from build123d import *

# Parameters (mm, degrees)
SKETCH_2_R                   = 2.5
SM_BASE_FLANGE_1_DEPTH       = 2
FILLET_1_R                   = 5
SM_EDGE_FLANGE_1_DEPTH       = 105
SM_EDGE_FLANGE_2_DEPTH       = 65
SM_START                     = 2
SM_EDGE_FLANGE_2_PROFILE_W   = 65
SM_EDGE_FLANGE_2_PROFILE_H   = 131
SM_EDGE_FLANGE_2_PROFILE_W_2 = 28
SM_EDGE_FLANGE_2_PROFILE_H_2 = 3
SM_EDGE_FLANGE_2_FLAT_DEPTH  = 2
SM_EDGE_FLANGE_3_DEPTH       = 105
SM_EDGE_FLANGE_3_PROFILE_W   = 9
SM_EDGE_FLANGE_3_PROFILE_H   = 9
SM_EDGE_FLANGE_3_FLAT_DEPTH  = 2
FILLET_3_R                   = 5
FILLET_4_R                   = 2
SM_EDGE_FLANGE_4_DEPTH       = 50
SM_EDGE_FLANGE_4_BEND_DEPTH  = 50
FILLET_2_R                   = 10


# Sheet-metal steps are written as plain solids
with BuildPart() as part:
    # Sketch 2 → Базовая кромка1 (new body)
    with BuildSketch(Plane(origin=(0, 0, 0), x_dir=(1, 0, 0), z_dir=(0, 1, 0))):
        Polygon((-90, -54), (-90, -86), (90, -86), (90, -66), (105, -66), (105, -34), (90, -34), (90, 34), (105, 34), (105, 66), (90, 66), (90, 86), (-90, 86), (-90, 54), (-75, 54), (-75, -54), align=None)
        with Locations(Location((-83, 80, 0), (0, 0, 270))):
            Circle(SKETCH_2_R, mode=Mode.SUBTRACT)
        with Locations(Location((-83, 60, 0), (0, 0, 270))):
            Circle(SKETCH_2_R, mode=Mode.SUBTRACT)
        with Locations(Location((98, 60, 0), (0, 0, 270))):
            Circle(SKETCH_2_R, mode=Mode.SUBTRACT)
        with Locations(Location((98, 40, 0), (0, 0, 270))):
            Circle(SKETCH_2_R, mode=Mode.SUBTRACT)
        with Locations(Location((98, -40, 0), (0, 0, 270))):
            Circle(SKETCH_2_R, mode=Mode.SUBTRACT)
        with Locations(Location((98, -60, 0), (0, 0, 270))):
            Circle(SKETCH_2_R, mode=Mode.SUBTRACT)
        with Locations(Location((-83, -60, 0), (0, 0, 270))):
            Circle(SKETCH_2_R, mode=Mode.SUBTRACT)
        with Locations(Location((-83, -80, 0), (0, 0, 270))):
            Circle(SKETCH_2_R, mode=Mode.SUBTRACT)
        with BuildLine():
            Line((-65, 15), (-65, -15))
            ThreePointArc((-65, -15), (-62.071067812, -22.071067812), (-55, -25))
            Line((-55, -25), (55, -25))
            ThreePointArc((55, -25), (62.071067812, -22.071067812), (65, -15))
            Line((65, -15), (65, 15))
            ThreePointArc((65, 15), (62.071067812, 22.071067812), (55, 25))
            Line((55, 25), (-55, 25))
            ThreePointArc((-55, 25), (-62.071067812, 22.071067812), (-65, 15))
        make_face(mode=Mode.SUBTRACT)
    extrude(amount=-SM_BASE_FLANGE_1_DEPTH)

    # Скругление1
    fillet_1_edges = [part.edges().sort_by_distance(p)[0] for p in [
        (105, -1, 66),
        (90, -1, 86),
        (-90, -1, 86),
        (-90, -1, 54),
        (-90, -1, -54),
        (-90, -1, -86),
        (90, -1, -86),
        (105, -1, -66),
        (105, -1, -34),
        (105, -1, 34),
    ]]
    fillet(fillet_1_edges, radius=FILLET_1_R)

    # Ребро-кромка1 section (across the edge) → Ребро-кромка1 (add)
    with BuildSketch(Plane(origin=(-78, 0, -52.5), x_dir=(1, 0, 0), z_dir=(0, 0, 1))):
        with BuildLine():
            Line((-2, 2), (-2, 96))
            Line((-2, 96), (0, 96))
            Line((0, 96), (0, 2))
            ThreePointArc((0, 2), (0.585786438, 0.585786438), (2, 0))
            Line((2, 0), (3, 0))
            Line((3, 0), (3, -2))
            Line((3, -2), (2, -2))
            ThreePointArc((2, -2), (-0.828427125, -0.828427125), (-2, 2))
        make_face()
    extrude(amount=SM_EDGE_FLANGE_1_DEPTH)

    # Ребро-кромка2 bend section (across the edge) → Ребро-кромка2 (add)
    with BuildSketch(Plane(origin=(92, 0, 32.5), x_dir=(-1, 0, 0), z_dir=(0, 0, -1))):
        with BuildLine():
            Line((-2, 2), (0, 2))
            ThreePointArc((0, 2), (0.585786438, 0.585786438), (2, 0))
            Line((2, 0), (2, -2))
            ThreePointArc((2, -2), (-0.828427125, -0.828427125), (-2, 2))
        make_face()
    extrude(amount=SM_EDGE_FLANGE_2_DEPTH)

    # Ребро-кромка2 profile (on flange) → Ребро-кромка2 flat (add)
    with BuildSketch(Plane(origin=(92, 0, 0), x_dir=(0, 0, -1), z_dir=(1, 0, 0)).offset(SM_START)):
        with Locations((0, 67.5)):
            Rectangle(SM_EDGE_FLANGE_2_PROFILE_W, SM_EDGE_FLANGE_2_PROFILE_H)
        with Locations((0, 127.5)):
            Rectangle(SM_EDGE_FLANGE_2_PROFILE_W_2, SM_EDGE_FLANGE_2_PROFILE_H_2, mode=Mode.SUBTRACT)
    extrude(amount=-SM_EDGE_FLANGE_2_FLAT_DEPTH)

    # Ребро-кромка3 bend section (across the edge) → Ребро-кромка3 (add)
    with BuildSketch(Plane(origin=(-80, 98, 52.5), x_dir=(0, -1, 0), z_dir=(0, 0, -1))):
        with BuildLine():
            Line((-2, 2), (0, 2))
            ThreePointArc((0, 2), (0.585786438, 0.585786438), (2, 0))
            Line((2, 0), (2, -2))
            ThreePointArc((2, -2), (-0.828427125, -0.828427125), (-2, 2))
        make_face()
    extrude(amount=SM_EDGE_FLANGE_3_DEPTH)

    # Ребро-кромка3 profile (on flange) → Ребро-кромка3 flat (add)
    with BuildSketch(Plane(origin=(-80, 98, 0), x_dir=(0, 0, -1), z_dir=(0, 1, 0)).offset(SM_START)):
        Polygon((-52.5, 8), (-52.5, 2), (52.5, 2), (52.5, 8), (12.5, 8), (12.5, 21), (-12.5, 21), (-12.5, 8), align=None)
        with Locations((0, 13)):
            Rectangle(SM_EDGE_FLANGE_3_PROFILE_W, SM_EDGE_FLANGE_3_PROFILE_H, mode=Mode.SUBTRACT)
    extrude(amount=-SM_EDGE_FLANGE_3_FLAT_DEPTH)

    # Скругление3
    fillet_3_edges = [part.edges().sort_by_distance(p)[0] for p in [
        (-88, 99, 52.5),
        (-88, 99, -52.5),
        (-101, 99, -12.5),
        (-101, 99, 12.5),
    ]]
    fillet(fillet_3_edges, radius=FILLET_3_R)

    # Скругление4
    fillet_4_edges = [part.edges().sort_by_distance(p)[0] for p in [
        (-88, 99, -12.5),
        (-88, 99, 12.5),
    ]]
    fillet(fillet_4_edges, radius=FILLET_4_R)

    # Ребро-кромка4 section (across the edge) → Ребро-кромка4 (add)
    with BuildSketch(Plane(origin=(-25, 0, 88), x_dir=(0, 0, -1), z_dir=(1, 0, 0))):
        with BuildLine():
            Line((-2, 2), (-2, 15))
            Line((-2, 15), (0, 15))
            Line((0, 15), (0, 2))
            ThreePointArc((0, 2), (0.585786438, 0.585786438), (2, 0))
            Line((2, 0), (2, -2))
            ThreePointArc((2, -2), (-0.828427125, -0.828427125), (-2, 2))
        make_face()
    extrude(amount=SM_EDGE_FLANGE_4_DEPTH)

    # Ребро-кромка4 section 2 (across the edge) → Ребро-кромка4 bend (add)
    with BuildSketch(Plane(origin=(25, 0, -88), x_dir=(0, 0, 1), z_dir=(-1, 0, 0))):
        with BuildLine():
            Line((-2, 2), (-2, 15))
            Line((-2, 15), (0, 15))
            Line((0, 15), (0, 2))
            ThreePointArc((0, 2), (0.585786438, 0.585786438), (2, 0))
            Line((2, 0), (2, -2))
            ThreePointArc((2, -2), (-0.828427125, -0.828427125), (-2, 2))
        make_face()
    extrude(amount=SM_EDGE_FLANGE_4_BEND_DEPTH)

    # Скругление2
    fillet_2_edges = [part.edges().sort_by_distance(p)[0] for p in [
        (93, 133, 32.5),
        (93, 133, -32.5),
        (-25, 15, 89),
        (25, 15, 89),
        (25, 15, -89),
        (-25, 15, -89),
    ]]
    fillet(fillet_2_edges, radius=FILLET_2_R)


solid = part.part
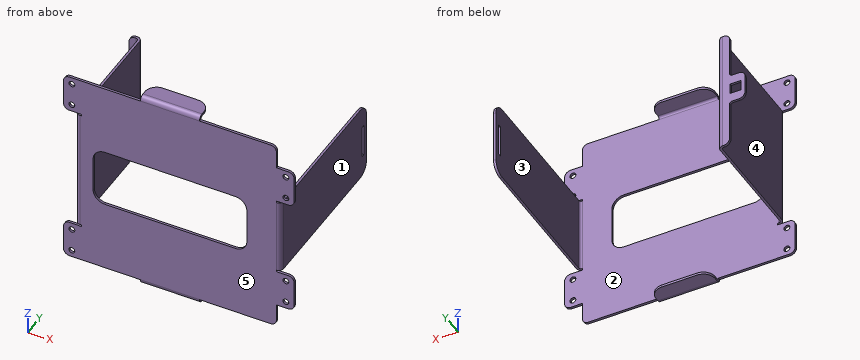
The model under review builds one solid part; all positions refer to its coordinate system, in mm. Face numbers are marked on the shaded views. A direction names the side the tool comes from. Give positions to 0.01 mm unless a question says otherwise; leave off trailing zeros. Write each loop counter-clockwise with the first axis right and the second up, starting at its lowest first coordinate (ties: lowest second). Pieces come first, ordered by that corner, then holes.
1. Tool access review of the marked faces 3, 4 and 5: name each direction out of +Z, -Z, +X, -X, +Y, -Y from which nothing blocks a thin tool from reaching the whole face with its end or side.
2. For P1, Ø1, axis at y = 96.5, z = 30, coming from the +X side; P2, Ø6.5, axis at x = -83, z = 80, coming from the -Y side; P3, Ø2, axis at y = -1, z = 71.5, coming from the +X side; P4, Ø15, axis at x = -90, z = -13.5, coming from the +Y side, all flat-tipped, find the tip position at first contact; note any pin that passes through.
3. Wall thickness on L1, parallel to X at y = -0.45, z = -60; L2, parallel to X at y = 81, z = 14.5; L3, parallel to Y at x = 41.5, z = -44: over which ranges is each line inside the solid? List them lowest first.
4. Add section B-B, the plane y = 88. Write out the cut boundary in (x, z), plus the area to 3 significant figures.
5. Add section A-A, the plane x = -44.5. Write out the cut boundary in (y, z), plus the area to 3 significant figures.
6. Draft analysis for pull direction Z (two halves, no side actions). For the marked faces 1 and 2, state which applies: +Z half, -Z half, draft (parallel to the pull), parting line (faces both ways), or undercut.
Worked answers:
1. face 3: +Z, -Z, +Y
1. face 4: +Z, -Z, -X, -Y
1. face 5: +Z, -Z, +X, -X, -Y
2. P1: stops at x = 94
2. P2: stops at y = -2
2. P3: stops at x = 90
2. P4: stops at y = 100
3. L1: x = -90 to -85.5, -80.5 to 95.5, 100.5 to 105
3. L2: x = -80 to -78, 92 to 94
3. L3: y = -2 to 0
4. outline: (-80, -52.5) - (-78, -52.5) - (-78, 52.5) - (-80, 52.5) - close; (92, -32.5) - (94, -32.5) - (94, 32.5) - (92, 32.5) - close
4. area: 340 mm2
5. outline: (-2, -86) - (0, -86) - (0, -25) - (-2, -25) - close; (-2, 25) - (0, 25) - (0, 86) - (-2, 86) - close
5. area: 244 mm2
6. face 1: draft
6. face 2: undercut
